The drawing under review shows one solid part. Ordinate dimensions are in mm from its lowest x, y, z. A direction names the side the tool comes from. Coordinates: 2 decimals unless noted, no trailing zeros. Write each loop counter-clockwise with the first axis right and the second up, starting at its lowest first coordinate (ties: lowest second). Pieces come first, ordered by that corner, then holes. Notation, with made-up numbers: (71.5, 7) - (126.5, 7) arc R24 cw to (126.5, 30) - close; hole circle Ø1 at (-4.75, 6). An arc over 180 degrees is marked (long way). Answer as CSV lines item,"result". Start each with the question number.
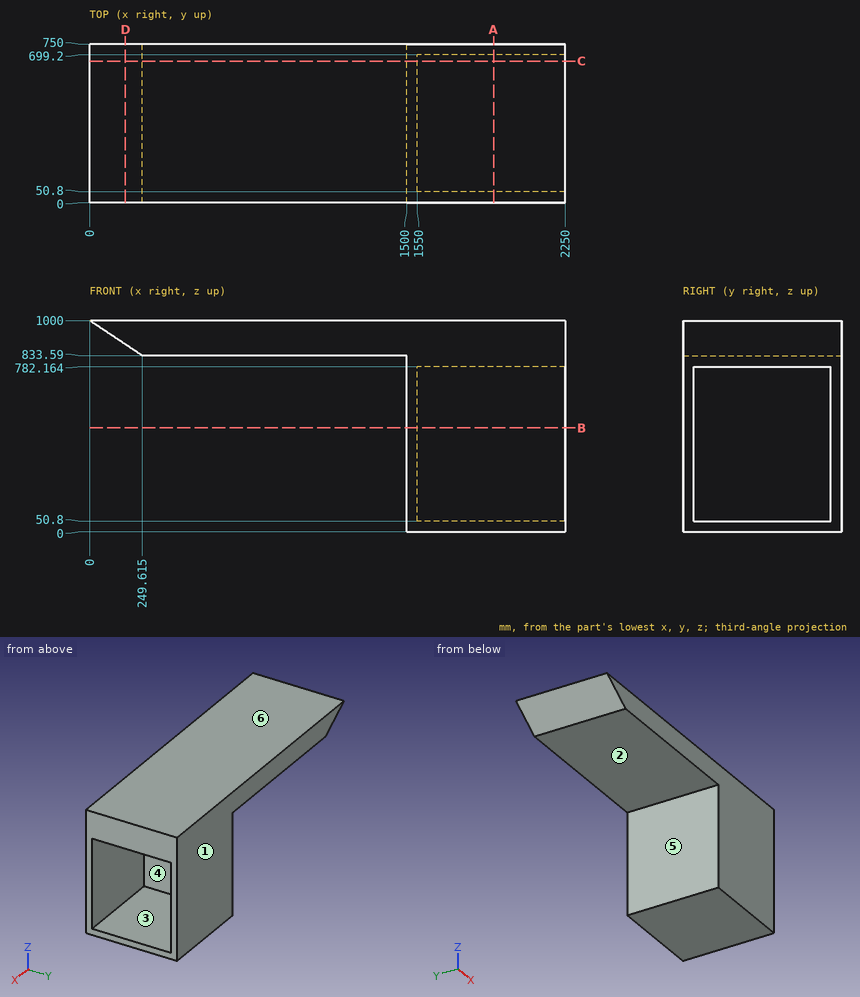
(1) For pin 1 (8 mm diameter, centred on y = 605, z = 643.5, fed in from -X); pin 2 (10 mm diameter, centred on y = 641.5, z = 252.5, fed in from +X); pin 3 (5 mm diameter, centred on x = 487, y = 563.5, fed in from -Z), all flat-tipped, find the tip position at first contact; note any pin that passes through.
(2) Add section D-D on x = 169.5. Give the boundary of the cut face in (y, z), then the cut area to 4 significant figures.
(3) For the marked faces 1, 2 and 3, list the 3-axis set-ups (+Z, -Z, +X, -X, +Y, -Y) from which the entire face can be reached by the end or side of a thin tool; tool diameter is ignored.
(4) Add section A-A on x = 1912. Give the boundary of the cut face in (y, z) (1 decimal).
(5) Add section B-B on z = 491.5. Give the boundary of the cut face in (x, y).
(6) Wall thickness on line 1 (Y direction, x = 1886, z = 65); line 2 (Z direction, x = 1629.5, y = 238.5) (1 decimal); line 3 (Z direction, x = 1074.5, y = 627): over which ranges is each line inside the solid? List them lowest first.
(7) Add section C-C on y = 669. Give the boundary of the cut face in (x, z) (1 decimal).
(8) The part is to be moulded in two halves that separate along Z. For the marked faces 4, 5 and 6, say which applies: released by +Z, released by -Z, zero draft, split by the parting line, or undercut.
Reported:
1,pin 1,"x = 1500"
1,pin 2,"x = 1550"
1,pin 3,"z = 833.59"
2,outline,"(0, 887) - (750, 887) - (750, 1000) - (0, 1000) - close"
2,area,"84,750 mm²"
3,face 1,"+Z, -Z, +X, -X, +Y"
3,face 2,"-Z, -X, +Y, -Y"
3,face 3,"+X"
4,outline,"(0, 0) - (750, 0) - (750, 1000) - (0, 1000) - close; hole (50.8, 50.8) - (699.2, 50.8) - (699.2, 782.2) - (50.8, 782.2) - close"
5,outline,"(1500, 0) - (2250, 0) - (2250, 50.8) - (1550, 50.8) - (1550, 699.2) - (2250, 699.2) - (2250, 750) - (1500, 750) - close"
6,line 1,"0 to 50.8, 699.2 to 750"
6,line 2,"0 to 50.8, 782.2 to 1000"
6,line 3,"833.59 to 1000"
7,outline,"(0, 1000) - (249.6, 833.6) - (1500, 833.6) - (1500, 0) - (2250, 0) - (2250, 50.8) - (1550, 50.8) - (1550, 782.2) - (2250, 782.2) - (2250, 1000) - close"
8,face 4,"undercut"
8,face 5,"zero draft"
8,face 6,"released by +Z"
